Part model, mm, in its own coordinate system. Give positions to 0.01 mm unless a question says otherwise; leave off trailing zeros. Order: outer loops, then holes, each group sorted by start corner. A loop starts at its lowest first (then second) coordinate and runs counter-clockwise, first axis right, second up. Notation, with made-up numbers: M 52,72.5 L 61,72.5 A22 ccw 61,84.5 Z; hole C 71.25,-26 d11. An arc over 180 degrees is marked long. One line per question, with ' | ' between items.
```python
from build123d import *

# Parameters (mm, degrees)
SKETCH2_R           = 5
BOSS_EXTRUDE1_DEPTH = 5


with BuildPart() as part:
    # Sketch2 → Boss-Extrude1 (new body)
    with BuildSketch(Plane(origin=(0, 0, 0), x_dir=(0, 1, 0), z_dir=(0, 0, 1))):
        with BuildLine():
            Line((-275, 12.5), (275, 12.5))
            ThreePointArc((275, 12.5), (287.5, 0), (275, -12.5))
            Line((275, -12.5), (-275, -12.5))
            ThreePointArc((-275, -12.5), (-287.5, 0), (-275, 12.5))
        make_face()
        with Locations(Location((-275, 0, 0), (0, 0, 270))):
            Circle(SKETCH2_R, mode=Mode.SUBTRACT)
        with Locations(Location((-206.25, 0, 0), (0, 0, 270))):
            Circle(SKETCH2_R, mode=Mode.SUBTRACT)
        with Locations(Location((-137.5, 0, 0), (0, 0, 270))):
            Circle(SKETCH2_R, mode=Mode.SUBTRACT)
        with Locations(Location((-68.75, 0, 0), (0, 0, 270))):
            Circle(SKETCH2_R, mode=Mode.SUBTRACT)
        with Locations(Location((0, 0, 0), (0, 0, 270))):
            Circle(SKETCH2_R, mode=Mode.SUBTRACT)
        with Locations(Location((68.75, 0, 0), (0, 0, 270))):
            Circle(SKETCH2_R, mode=Mode.SUBTRACT)
        with Locations(Location((137.5, 0, 0), (0, 0, 270))):
            Circle(SKETCH2_R, mode=Mode.SUBTRACT)
        with Locations(Location((206.25, 0, 0), (0, 0, 270))):
            Circle(SKETCH2_R, mode=Mode.SUBTRACT)
        with Locations(Location((275, 0, 0), (0, 0, 270))):
            Circle(SKETCH2_R, mode=Mode.SUBTRACT)
    extrude(amount=BOSS_EXTRUDE1_DEPTH)


solid = part.part
```
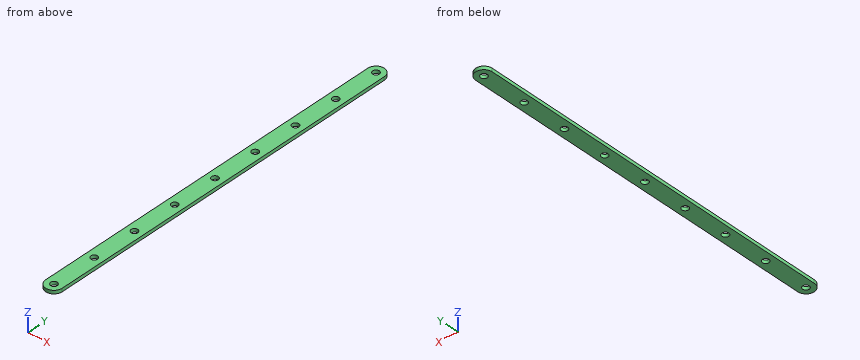
1. Slice it at B-B on z = 2.9. Give the number of separate pieces and of enclosed holes in the cut face, then the cut area to 3 significant figures.
Worked out:
separate pieces: 1 | enclosed holes: 9 | area: 13,500 mm2
2. Drop a flat-ended pin along its axis: pin 1 (8 mm diameter, centred on x = 0, y = 68.75, fed in from -Z). Give the stop position or say it passes through.
Worked out:
pin 1: passes through
3. Slice it at A-A on y = -68.75. Give the cut face in (x, z), then the cut area to 3 significant figures.
Worked out:
outline: M -12.5,0 L -5,0 L -5,5 L -12.5,5 Z; M 5,0 L 12.5,0 L 12.5,5 L 5,5 Z | area: 75.0 mm2
4. Probe L1, parallel to Y at x = -5.5, z = 3.15; L2, parallel to Y at x = -6.25, z = 4.25. List the from-to ranges inside material, lowest first. Write a range as from..to.
Worked out:
L1: y = -286.22..286.22 | L2: y = -285.83..285.83
